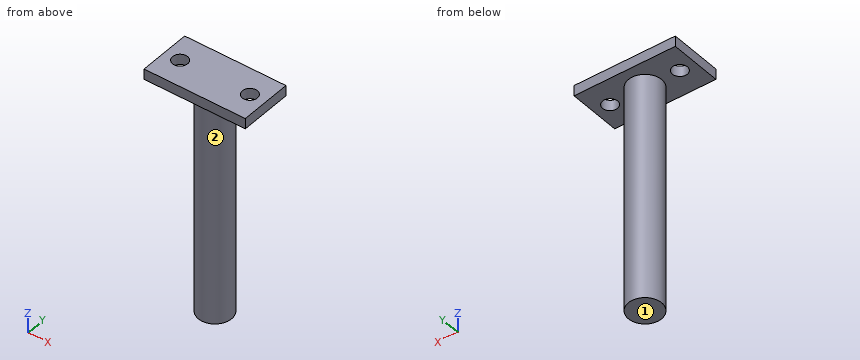
from build123d import *

# Parameters (mm, degrees)
SKETCH1_W                = 29
SKETCH1_H                = 15
SKETCH1_R                = 2.15
SKETCH1_R_2              = 4.75
BOSS_EXTRUDE1_DEPTH      = 3
SKETCH1_3_R              = 4.75
BOSS_EXTRUDE2_DEPTH      = 3
BOSS_EXTRUDE2_DEPTH_BACK = 65.1


with BuildPart() as part:
    # Sketch1 → Boss-Extrude1 (new body)
    with BuildSketch(Plane.XY):
        with Locations((-13.13286664, 8.093964388)):
            Rectangle(SKETCH1_W, SKETCH1_H)
        with Locations((-23.13286664, 8.093964388)):
            Circle(SKETCH1_R, mode=Mode.SUBTRACT)
        with Locations((-13.140365172, 8.093964388)):
            Circle(SKETCH1_R_2, mode=Mode.SUBTRACT)
        with Locations((-3.13286664, 8.093964388)):
            Circle(SKETCH1_R, mode=Mode.SUBTRACT)
    extrude(amount=BOSS_EXTRUDE1_DEPTH)

    # Sketch1<3> → Boss-Extrude2 (add, two sides)
    with BuildSketch(Plane.XY) as boss_extrude2_sk:
        with Locations((-13.140365172, 8.093964388)):
            Circle(SKETCH1_3_R)
    extrude(amount=BOSS_EXTRUDE2_DEPTH)
    extrude(boss_extrude2_sk.sketch, amount=-BOSS_EXTRUDE2_DEPTH_BACK)


solid = part.part
Geometry check sheet. Reference: the model listing, model coordinates, mm. Face numbers are marked on the shaded views. A direction names the side the tool comes from. Give positions to 0.01 mm unless a question says otherwise; leave off trailing zeros. Write each loop counter-clockwise with the first axis right and the second up, starting at its lowest first coordinate (ties: lowest second). Pieces come first, ordered by that corner, then holes. Notation, with made-up numbers: M -7.75,73.5 L 27.25,73.5 A21 ccw 27.25,79.5 Z; hole C -10,-30.75 d4. An arc over 180 degrees is marked long. Answer as CSV lines item,"result". Start each with the question number.
Q1. Section check D-D, the plane z = -19.5. Record the cut outline in (x, y), then the cut area to 3 significant figures.
Q2. Tool access check on the marked faces 1 and 2. Record the directions out of +Z, -Z, +X, -X, +Y, -Y that give a thin tool (end or side, any length) a straight path to the whole face; none if there is none.
Q3. Section check C-C, the plane y = 14. Record the cut outline in (x, z).
Q4. Section check A-A, the plane y = 7. Record the cut outline in (x, z).
Q5. Go/stop test with flat-tipped pins: pin 1 (6 mm diameter, centred on y = 3, z = -41.5, fed in from +X); pin 2 (1.5 mm diameter, centred on y = 9.5, z = -55, fed in from -X). Record where each tip stops, or that it passes through.
Q6. Section check B-B, the plane x = -24. Record the cut outline in (y, z), then the cut area to 3 significant figures.
Q7. Material ranges on L1, parallel to X at y = 8, z = -18.5; L2, parallel to Z at x = -19.5, y = 14.5; L3, parallel to X at y = 9.75, z = -14, recorded low to high.
Geometry says:
1,outline,"C -13.14,8.09 d9.5"
1,area,"70.9 mm^2"
2,face 1,"-Z, +X, -X, +Y, -Y"
2,face 2,"-Z"
3,outline,"M -27.63,0 L 1.37,0 L 1.37,3 L -27.63,3 Z"
4,outline,"M -27.63,0 L -24.98,0 L -24.98,3 L -27.63,3 Z; M -21.28,0 L -17.76,0 L -17.76,-65.1 L -8.52,-65.1 L -8.52,0 L -4.98,0 L -4.98,3 L -21.28,3 Z; M -1.28,0 L 1.37,0 L 1.37,3 L -1.28,3 Z"
5,pin 1,"x = -8.88"
5,pin 2,"x = -17.84"
6,outline,"M 0.59,0 L 6.13,0 L 6.13,3 L 0.59,3 Z; M 10.06,0 L 15.59,0 L 15.59,3 L 10.06,3 Z"
6,area,"33.2 mm^2"
7,L1,"-17.89 to -8.39"
7,L2,"0 to 3"
7,L3,"-17.59 to -8.69"
